Could you check a few things on this drawing? It's one solid part, dimensions in mm from its lowest x, y, z. A direction names the side the tool comes from. Round coordinates to 2 decimals unless told otherwise and drop trailing zeros. Write each loop counter-clockwise with the first axis right and the second up, starting at its lowest first coordinate (ties: lowest second). Pieces come first, ordered by that corner, then holes. Notation, with made-up numbers: M 47.5,44.5 L 88.5,44.5 A5 ccw 88.5,50.5 Z; hole C 82,84.5 d9. An arc over 180 degrees is marked long. One line per item, written item: value. Start each with the question number.
(1) Thinking about a two-plate mould opening in Y: for the marked faces 4, 5 and 6, which applies, released by +Y, released by -Y, zero draft, split by the parting line, or undercut?
(2) Which directions (+Z, -Z, +X, -X, +Y, -Y) give clear straight access to the entire face, cutting with the end or side of a thin tool? Please do the marked faces 1, 2 and 3.
(3) I want a section at D-D on z = 1.2. Please give me the cut outline in (x, y).
(4) If I drill on L1, parallel to Y at x = 2.56, z = 1.4; L2, parallel to X at y = 11, z = 0.4; L3, parallel to Y at x = 13, z = 1.55, over which ranges is the centre line in solid material (lowest first)?
(5) I want a section at A-A on x = 10. Please give me the cut outline in (y, z), and give its area (3 significant figures).
(6) I'm going to push a flat-ended pin straight in: pin 1 Ø1.5 at (x, z) = (13.5, 1.5) entering from -Y. Where does the tip first touch, or does it pass through?
(7) I want a section at B-B on y = 2.75. Please give me the cut outline in (x, z).
(8) I want a section at C-C on x = 20.44. Please give me the cut outline in (y, z).
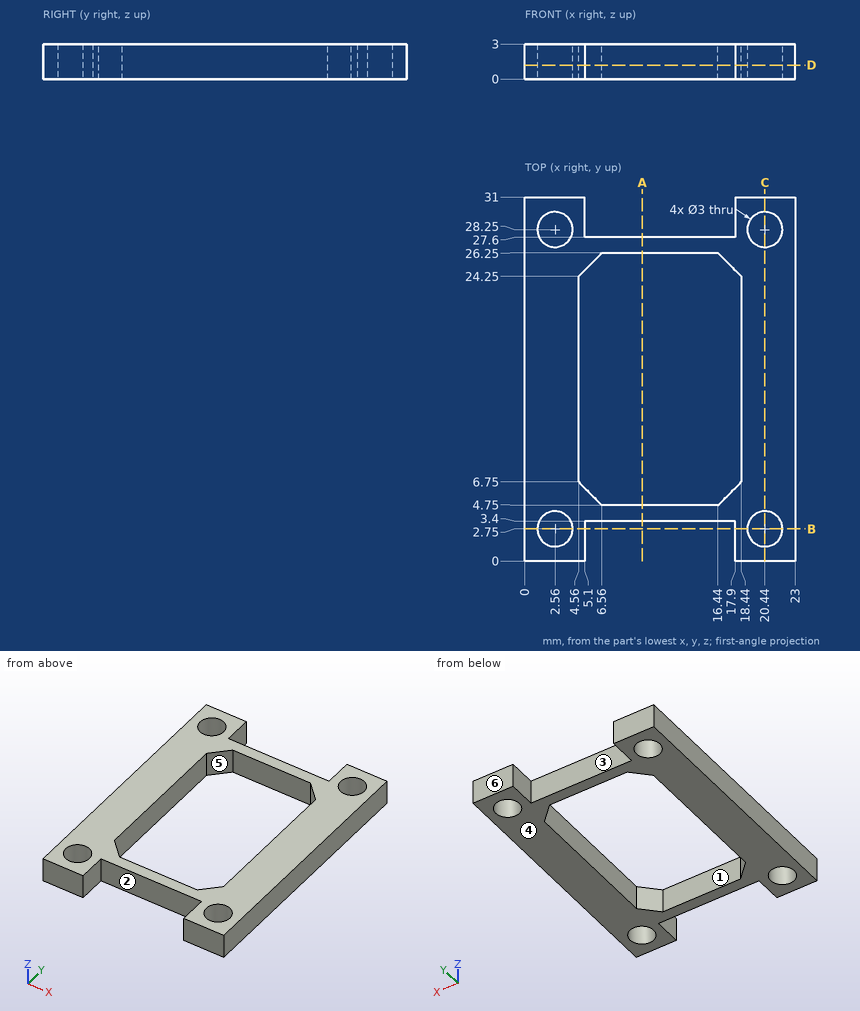
Found:
1. face 4: zero draft
1. face 5: undercut
1. face 6: released by +Y
2. face 1: +Z, -Z
2. face 2: +Z, -Z, -Y
2. face 3: +Z, -Z, +Y
3. outline: M 0,0 L 5.1,0 L 5.1,3.4 L 17.9,3.4 L 17.9,0 L 23,0 L 23,31 L 17.9,31 L 17.9,27.6 L 5.1,27.6 L 5.1,31 L 0,31 Z; hole C 2.56,2.75 d3; hole C 2.56,28.25 d3; hole M 4.56,6.75 L 6.56,4.75 L 16.44,4.75 L 18.44,6.75 L 18.44,24.25 L 16.44,26.25 L 6.56,26.25 L 4.56,24.25 Z; hole C 20.44,2.75 d3; hole C 20.44,28.25 d3
4. L1: y = 0 to 1.25, 4.25 to 26.75, 29.75 to 31
4. L2: x = 0 to 4.56, 18.44 to 23
4. L3: y = 3.4 to 4.75, 26.25 to 27.6
5. outline: M 3.4,0 L 4.75,0 L 4.75,3 L 3.4,3 Z; M 26.25,0 L 27.6,0 L 27.6,3 L 26.25,3 Z
5. area: 8.10 mm²
6. pin 1: stops at y = 3.4
7. outline: M 0,0 L 1.06,0 L 1.06,3 L 0,3 Z; M 4.06,0 L 5.1,0 L 5.1,3 L 4.06,3 Z; M 17.9,0 L 18.94,0 L 18.94,3 L 17.9,3 Z; M 21.94,0 L 23,0 L 23,3 L 21.94,3 Z
8. outline: M 0,0 L 1.25,0 L 1.25,3 L 0,3 Z; M 4.25,0 L 26.75,0 L 26.75,3 L 4.25,3 Z; M 29.75,0 L 31,0 L 31,3 L 29.75,3 Z
